Could you check a few things on this model? Use its own coordinates, in mm. A direction names the side the tool comes from. Give positions to 0.01 mm unless a question says otherwise; leave off trailing zeros. Loops run counter-clockwise (first coordinate to the right, second up) from the corner with the lowest first, then second, coordinate; pieces in that order, holes last. Notation, with made-up numbers: M 54,59.5 L 66,59.5 A20 cw 66,91.5 Z; hole C 20.5,85 d2. An arc over 180 degrees is marked long. Answer in a Markdown table with one row per item. Add a question column.
Autodesk Inventor part; units mm, degrees
ref_plane "YZ Plane" through (0, 0, 0) normal (1, 0, 0) x (0, 1, 0)
ref_plane "XZ Plane" through (0, 0, 0) normal (0, 1, 0) x (-1, 0, 0)
ref_plane "XY Plane" through (0, 0, 0) normal (0, 0, 1) x (1, 0, 0)
sketch "Sketch1" plane through (0, 0, 0) normal (1, 0, 0) x (0, 1, 0)
  line L0 (0, 0) -> (0, -40)
  line L1 (0, -40) -> (19, -40)
  line L2 (19, -40) -> (19, -38)
  line L3 (0, 0) -> (19, 0)
  line L4 (19, 0) -> (19, -2)
  line L5 (0, -20) -> (2, -20) construction
  line L6 (19, -2) -> (2, -2)
  line L7 (2, -2) -> (2, -38)
  line L8 (2, -38) -> (19, -38)
  dimension "d0" = 40
  dimension "d1" = 19
  dimension "d2" = 2
  dimension "d3" = 2
  dimension "d4" = 2
extrude "Extrusion1" add sketch "Sketch1" along normal blind 355.6
sketch "Sketch2" plane through (0, 2, -2) normal (0, 0, -1) x (-1, 0, 0)
  circle A0 centre (-13.8784, 10.3) radius 3.175
  point P0 (0, -2)
extrude "Extrusion2" cut sketch "Sketch2" against normal blind 25.4
sketch "Sketch3" plane through (0, 2, -2) normal (0, 0, -1) x (-1, 0, 0)
  circle A0 centre (-13.8784, 10.3) radius 3.175
  line L0 (-355.6, 0) -> (-355.6, 17)
  line L1 (0, 17) -> (-355.6, 17)
  circle A1 centre (-37.4708, 10.3) radius 3.175
  circle A2 centre (-177.8, 10.3) radius 3.175
  circle A3 centre (-340.3166, 10.3) radius 3.175
  point P0 (0, -2)
  dimension "d9" = 6.35
  dimension "d10" = 6.35
  dimension "d11" = 6.35
extrude "Extrusion3" cut sketch "Sketch3" against normal blind 25.4 contours A1 | A2 | A3
sketch "Sketch4" plane through (0, 0, -40) normal (0, 0, -1) x (-1, 0, 0)
  circle A0 centre (-348.1, 9.62) radius 3.175
  circle A1 centre (-7.5, 9.62) radius 3.175
extrude "Extrusion4" cut sketch "Sketch4" against normal blind 25.4
properties part number "26in C-Channel (TopPlate Supports)" material "Aluminum 6061"
Item 1: I need wall thicknesses on L1, parallel to Z at x = 53.5, y = 5; L2, parallel to Y at x = 348.1, z = -39.35 (3 decimals); L3, parallel to Y at x = 313.5, z = -14.5. Which ranges of each line are inside material? Lowest first, please.
Item 2: Suppose I cut it at B-B (z = -18). List the corners of the cut face in (x, y) for me.
Item 3: Suppose I cut it at C-C (x = 237). List the corners of the cut face in (y, z) for me, then the cut area to 3 significant figures.
Item 4: For P1, Ø5, axis at x = 348.1, y = 9.62, coming from the -Z side; P2, Ø12, axis at x = 281, z = -29.5, coming from the +Y side; P3, Ø5, axis at x = 13.88, y = 12.3, coming from the +Z side, each with a flat end and sliding along its axis, tell me the tip position at first contact or that it passes through.
Item 5: If we mould it in two halves opening along Z, with no side actions, what happens to faces 1 (the face through (175, 10, -38)), 2 (the face through (175, 9, -2)), 3 (the face through (180.97, 12.44, -1.01)), 4 (the face through (175, 9, -40))? For each: +Z half, -Z half, draft (parallel to the pull), parting line (faces both ways), or undercut.
Item 6: Suppose I cut it at A-A (x = 177.8). List the corners of the cut face in (y, z) for me (3 decimals), then the cut area to 3 significant figures.
Item 7: For faces 5 (the face through (8.19, 6.52, -39.01)), 6 (the face through (0, 1.7, -19.9)), 7 (the face through (175, 2, -20)), 8 (the face through (175, 9, 0)), 9 (the face through (14.57, 9.2, -1.01)), which set-ups out of +Z, -Z, +X, -X, +Y, -Y let a thin tool reach every point of the face, with its end or its side?
Values found:
| question | item | result |
|---|---|---|
| 1 | L1 | -40 to -38, -2 to 0 |
| 1 | L2 | 0 to 6.445, 12.795 to 19 |
| 1 | L3 | 0 to 2 |
| 2 | outline | M 0,0 L 355.6,0 L 355.6,2 L 0,2 Z |
| 3 | outline | M 0,-40 L 19,-40 L 19,-38 L 2,-38 L 2,-2 L 19,-2 L 19,0 L 0,0 Z |
| 3 | area | 148 mm² |
| 4 | P1 | z = -2 |
| 4 | P2 | y = 2 |
| 4 | P3 | z = -38 |
| 5 | face 1 | undercut |
| 5 | face 2 | undercut |
| 5 | face 3 | draft |
| 5 | face 4 | -Z half |
| 6 | outline | M 0,-40 L 19,-40 L 19,-38 L 2,-38 L 2,-2 L 9.125,-2 L 9.125,0 L 0,0 Z; M 15.475,-2 L 19,-2 L 19,0 L 15.475,0 Z |
| 6 | area | 135 mm² |
| 7 | face 5 | -Z |
| 7 | face 6 | +Z, -Z, -X, +Y, -Y |
| 7 | face 7 | +X, -X, +Y |
| 7 | face 8 | +Z, +X, -X, +Y, -Y |
| 7 | face 9 | +Z |
